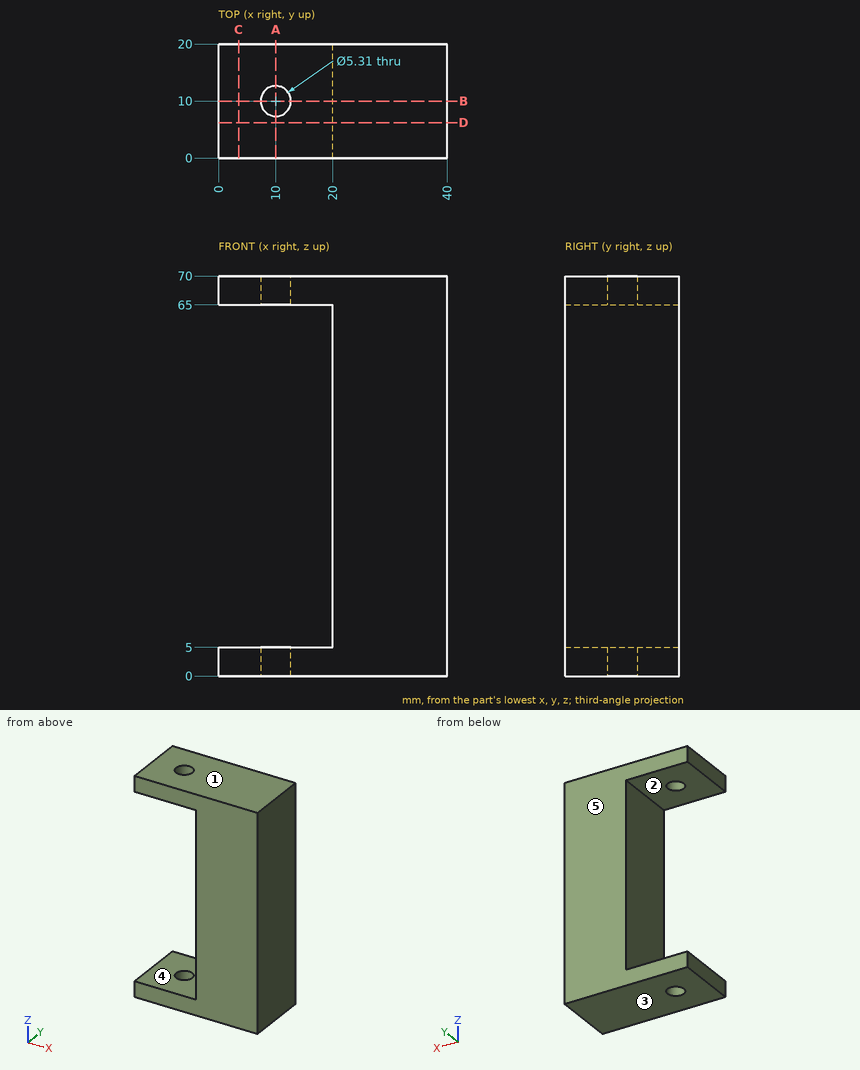
For this review, use the dimensioned drawing (mm, ordinates from the lowest corner) and the shaded views. A direction names the side the tool comes from. Give positions to 0.01 mm unless a question says otherwise; leave off trailing zeros. Order: outer loops, then holes, each group sorted by start corner. A loop starts at its lowest first (then second) coordinate and runs counter-clockwise, first axis right, second up. Notation, with made-up numbers: (82, 83) - (135, 83) arc R19 cw to (135, 94) - close; hole circle Ø10 at (24, 8.25). An arc over 180 degrees is marked (long way). Write item = value, one per line. Start each with the question number.
Q1. We need section A-A on x = 10. State the section outline as (y, z) points (3 decimals).
Q2. Tool access review of the marked faces 1 and 2: name each direction out of +Z, -Z, +X, -X, +Y, -Y from which nothing blocks a thin tool from reaching the whole face with its end or side.
Q3. Mouldability with a two-part tool opening along Z and no side actions: class the marked faces 3, 4 and 5 as released by +Z, released by -Z, zero draft, split by the parting line, or undercut.
Q4. We need section C-C on x = 3.5. State the section outline as (y, z) points.
Q5. To check wall thickness, follow L1, parallel to Y at x = 10, z = 1.7 (3 decimals); L2, parallel to Z at x = 18, y = 15.75; L3, parallel to X at y = 18.5, z = 53.5. State the ranges of each line that lie inside material, in increasing order. Write a range as from..to.
Q6. We need section D-D on y = 6.25. State the section outline as (x, z) points.
Q7. Clearance check with flat-ended pins moving along their axes: pin 1 Ø10 at (y, z) = (13.5, 38.5) entering from -X; pin 2 Ø4 at (x, y) = (10, 10) entering from -Z. State where each tip first meets the part, or that it passes through.
Q8. We need section B-B on y = 10. State the section outline as (x, z) points (3 decimals).
Working result:
q1.outline = (0, 0) - (7.345, 0) - (7.345, 5) - (0, 5) - close; (0, 65) - (7.345, 65) - (7.345, 70) - (0, 70) - close; (12.655, 0) - (20, 0) - (20, 5) - (12.655, 5) - close; (12.655, 65) - (20, 65) - (20, 70) - (12.655, 70) - close
q2.face_1 = +Z, +X, -X, +Y, -Y
q2.face_2 = -X, +Y, -Y
q3.face_3 = released by -Z
q3.face_4 = undercut
q3.face_5 = zero draft
q4.outline = (0, 0) - (20, 0) - (20, 5) - (0, 5) - close; (0, 65) - (20, 65) - (20, 70) - (0, 70) - close
q5.L1 = 0..7.345, 12.655..20
q5.L2 = 0..5, 65..70
q5.L3 = 20..40
q6.outline = (0, 0) - (40, 0) - (40, 70) - (0, 70) - (0, 65) - (20, 65) - (20, 5) - (0, 5) - close
q7.pin_1 = 20
q7.pin_2 = through
q8.outline = (0, 0) - (7.345, 0) - (7.345, 5) - (0, 5) - close; (0, 65) - (7.345, 65) - (7.345, 70) - (0, 70) - close; (12.655, 0) - (40, 0) - (40, 70) - (12.655, 70) - (12.655, 65) - (20, 65) - (20, 5) - (12.655, 5) - close
